```python
from build123d import *

# Parameters (mm, degrees)
CROQUIS2_W              = 180
CROQUIS2_H              = 90
SALIENTE_EXTRUIR1_DEPTH = 4
REDONDEO1_R             = 10
CORTAR_EXTRUIR1_REACH   = 102.703
CROQUIS8_R              = 2
CORTAR_EXTRUIR2_REACH   = 102.703
CROQUIS4_R              = 4
CROQUIS9_R              = 2
CORTAR_EXTRUIR3_DEPTH   = 101.702532242


with BuildPart() as part:
    # Croquis2 → Saliente-Extruir1 (new body)
    with BuildSketch(Plane(origin=(0, 0, 0), x_dir=(1, 0, 0), z_dir=(0, 1, 0))):
        Rectangle(CROQUIS2_W, CROQUIS2_H)
    extrude(amount=SALIENTE_EXTRUIR1_DEPTH)

    # Redondeo1
    redondeo1_edges = [part.edges().sort_by_distance(p)[0] for p in [
        (90, 2, 45),
        (-90, 2, 45),
        (-90, 2, -45),
        (90, 2, -45),
    ]]
    fillet(redondeo1_edges, radius=REDONDEO1_R)

    # Croquis8 → Cortar-Extruir1 (cut, up to next)
    with BuildSketch(Plane(origin=(0, 4, 0), x_dir=(1, 0, 0), z_dir=(0, 1, 0)), mode=Mode.PRIVATE) as cortar_extruir1_sk1:
        with Locations(Location((-47, 0, 0), (0, 0, 270))):
            Circle(CROQUIS8_R)
    cortar_extruir1_tool1 = extrude(cortar_extruir1_sk1.sketch, amount=-CORTAR_EXTRUIR1_REACH, mode=Mode.PRIVATE) & part.part
    # Croquis8 → Cortar-Extruir1 (cut, up to next)
    with BuildSketch(Plane(origin=(0, 4, 0), x_dir=(1, 0, 0), z_dir=(0, 1, 0)), mode=Mode.PRIVATE) as cortar_extruir1_sk2:
        with Locations(Location((-77, 0, 0), (0, 0, 270))):
            Circle(CROQUIS8_R)
    cortar_extruir1_tool2 = extrude(cortar_extruir1_sk2.sketch, amount=-CORTAR_EXTRUIR1_REACH, mode=Mode.PRIVATE) & part.part
    # Croquis8 → Cortar-Extruir1 (cut, up to next)
    with BuildSketch(Plane(origin=(0, 4, 0), x_dir=(1, 0, 0), z_dir=(0, 1, 0)), mode=Mode.PRIVATE) as cortar_extruir1_sk3:
        with Locations(Location((77, 0, 0), (0, 0, 90))):
            Circle(CROQUIS8_R)
    cortar_extruir1_tool3 = extrude(cortar_extruir1_sk3.sketch, amount=-CORTAR_EXTRUIR1_REACH, mode=Mode.PRIVATE) & part.part
    # Croquis8 → Cortar-Extruir1 (cut, up to next)
    with BuildSketch(Plane(origin=(0, 4, 0), x_dir=(1, 0, 0), z_dir=(0, 1, 0)), mode=Mode.PRIVATE) as cortar_extruir1_sk4:
        with Locations(Location((47, 0, 0), (0, 0, 90))):
            Circle(CROQUIS8_R)
    cortar_extruir1_tool4 = extrude(cortar_extruir1_sk4.sketch, amount=-CORTAR_EXTRUIR1_REACH, mode=Mode.PRIVATE) & part.part
    # Croquis8 → Cortar-Extruir1 (cut, up to next)
    with BuildSketch(Plane(origin=(0, 4, 0), x_dir=(1, 0, 0), z_dir=(0, 1, 0)), mode=Mode.PRIVATE) as cortar_extruir1_sk5:
        with Locations(Location((-77, 15.5, 0), (0, 0, 270))):
            Circle(CROQUIS8_R)
    cortar_extruir1_tool5 = extrude(cortar_extruir1_sk5.sketch, amount=-CORTAR_EXTRUIR1_REACH, mode=Mode.PRIVATE) & part.part
    # Croquis8 → Cortar-Extruir1 (cut, up to next)
    with BuildSketch(Plane(origin=(0, 4, 0), x_dir=(1, 0, 0), z_dir=(0, 1, 0)), mode=Mode.PRIVATE) as cortar_extruir1_sk6:
        with Locations(Location((-47, 15.5, 0), (0, 0, 270))):
            Circle(CROQUIS8_R)
    cortar_extruir1_tool6 = extrude(cortar_extruir1_sk6.sketch, amount=-CORTAR_EXTRUIR1_REACH, mode=Mode.PRIVATE) & part.part
    # Croquis8 → Cortar-Extruir1 (cut, up to next)
    with BuildSketch(Plane(origin=(0, 4, 0), x_dir=(1, 0, 0), z_dir=(0, 1, 0)), mode=Mode.PRIVATE) as cortar_extruir1_sk7:
        with Locations(Location((-77, -15.5, 0), (0, 0, 90))):
            Circle(CROQUIS8_R)
    cortar_extruir1_tool7 = extrude(cortar_extruir1_sk7.sketch, amount=-CORTAR_EXTRUIR1_REACH, mode=Mode.PRIVATE) & part.part
    # Croquis8 → Cortar-Extruir1 (cut, up to next)
    with BuildSketch(Plane(origin=(0, 4, 0), x_dir=(1, 0, 0), z_dir=(0, 1, 0)), mode=Mode.PRIVATE) as cortar_extruir1_sk8:
        with Locations(Location((-47, -15.5, 0), (0, 0, 90))):
            Circle(CROQUIS8_R)
    cortar_extruir1_tool8 = extrude(cortar_extruir1_sk8.sketch, amount=-CORTAR_EXTRUIR1_REACH, mode=Mode.PRIVATE) & part.part
    # Croquis8 → Cortar-Extruir1 (cut, up to next)
    with BuildSketch(Plane(origin=(0, 4, 0), x_dir=(1, 0, 0), z_dir=(0, 1, 0)), mode=Mode.PRIVATE) as cortar_extruir1_sk9:
        with Locations(Location((47, -15.5, 0), (0, 0, 270))):
            Circle(CROQUIS8_R)
    cortar_extruir1_tool9 = extrude(cortar_extruir1_sk9.sketch, amount=-CORTAR_EXTRUIR1_REACH, mode=Mode.PRIVATE) & part.part
    # Croquis8 → Cortar-Extruir1 (cut, up to next)
    with BuildSketch(Plane(origin=(0, 4, 0), x_dir=(1, 0, 0), z_dir=(0, 1, 0)), mode=Mode.PRIVATE) as cortar_extruir1_sk10:
        with Locations(Location((77, -15.5, 0), (0, 0, 270))):
            Circle(CROQUIS8_R)
    cortar_extruir1_tool10 = extrude(cortar_extruir1_sk10.sketch, amount=-CORTAR_EXTRUIR1_REACH, mode=Mode.PRIVATE) & part.part
    # Croquis8 → Cortar-Extruir1 (cut, up to next)
    with BuildSketch(Plane(origin=(0, 4, 0), x_dir=(1, 0, 0), z_dir=(0, 1, 0)), mode=Mode.PRIVATE) as cortar_extruir1_sk11:
        with Locations(Location((77, 15.5, 0), (0, 0, 90))):
            Circle(CROQUIS8_R)
    cortar_extruir1_tool11 = extrude(cortar_extruir1_sk11.sketch, amount=-CORTAR_EXTRUIR1_REACH, mode=Mode.PRIVATE) & part.part
    # Croquis8 → Cortar-Extruir1 (cut, up to next)
    with BuildSketch(Plane(origin=(0, 4, 0), x_dir=(1, 0, 0), z_dir=(0, 1, 0)), mode=Mode.PRIVATE) as cortar_extruir1_sk12:
        with Locations(Location((47, 15.5, 0), (0, 0, 90))):
            Circle(CROQUIS8_R)
    cortar_extruir1_tool12 = extrude(cortar_extruir1_sk12.sketch, amount=-CORTAR_EXTRUIR1_REACH, mode=Mode.PRIVATE) & part.part
    add(cortar_extruir1_tool1.solids().sort_by_distance((-47, 4, 0))[0], mode=Mode.SUBTRACT)
    add(cortar_extruir1_tool2.solids().sort_by_distance((-77, 4, 0))[0], mode=Mode.SUBTRACT)
    add(cortar_extruir1_tool3.solids().sort_by_distance((77, 4, 0))[0], mode=Mode.SUBTRACT)
    add(cortar_extruir1_tool4.solids().sort_by_distance((47, 4, 0))[0], mode=Mode.SUBTRACT)
    add(cortar_extruir1_tool5.solids().sort_by_distance((-77, 4, -15.5))[0], mode=Mode.SUBTRACT)
    add(cortar_extruir1_tool6.solids().sort_by_distance((-47, 4, -15.5))[0], mode=Mode.SUBTRACT)
    add(cortar_extruir1_tool7.solids().sort_by_distance((-77, 4, 15.5))[0], mode=Mode.SUBTRACT)
    add(cortar_extruir1_tool8.solids().sort_by_distance((-47, 4, 15.5))[0], mode=Mode.SUBTRACT)
    add(cortar_extruir1_tool9.solids().sort_by_distance((47, 4, 15.5))[0], mode=Mode.SUBTRACT)
    add(cortar_extruir1_tool10.solids().sort_by_distance((77, 4, 15.5))[0], mode=Mode.SUBTRACT)
    add(cortar_extruir1_tool11.solids().sort_by_distance((77, 4, -15.5))[0], mode=Mode.SUBTRACT)
    add(cortar_extruir1_tool12.solids().sort_by_distance((47, 4, -15.5))[0], mode=Mode.SUBTRACT)

    # Croquis4 → Cortar-Extruir2 (cut, up to next)
    with BuildSketch(Plane(origin=(0, 4, 0), x_dir=(1, 0, 0), z_dir=(0, 1, 0)), mode=Mode.PRIVATE) as cortar_extruir2_sk1:
        with Locations(Location((-80, 35, 0), (0, 0, 270))):
            Circle(CROQUIS4_R)
    cortar_extruir2_tool1 = extrude(cortar_extruir2_sk1.sketch, amount=-CORTAR_EXTRUIR2_REACH, mode=Mode.PRIVATE) & part.part
    # Croquis4 → Cortar-Extruir2 (cut, up to next)
    with BuildSketch(Plane(origin=(0, 4, 0), x_dir=(1, 0, 0), z_dir=(0, 1, 0)), mode=Mode.PRIVATE) as cortar_extruir2_sk2:
        with Locations(Location((-80, -35, 0), (0, 0, 270))):
            Circle(CROQUIS4_R)
    cortar_extruir2_tool2 = extrude(cortar_extruir2_sk2.sketch, amount=-CORTAR_EXTRUIR2_REACH, mode=Mode.PRIVATE) & part.part
    # Croquis4 → Cortar-Extruir2 (cut, up to next)
    with BuildSketch(Plane(origin=(0, 4, 0), x_dir=(1, 0, 0), z_dir=(0, 1, 0)), mode=Mode.PRIVATE) as cortar_extruir2_sk3:
        with Locations(Location((80, -35, 0), (0, 0, 90))):
            Circle(CROQUIS4_R)
    cortar_extruir2_tool3 = extrude(cortar_extruir2_sk3.sketch, amount=-CORTAR_EXTRUIR2_REACH, mode=Mode.PRIVATE) & part.part
    # Croquis4 → Cortar-Extruir2 (cut, up to next)
    with BuildSketch(Plane(origin=(0, 4, 0), x_dir=(1, 0, 0), z_dir=(0, 1, 0)), mode=Mode.PRIVATE) as cortar_extruir2_sk4:
        with Locations(Location((80, 35, 0), (0, 0, 90))):
            Circle(CROQUIS4_R)
    cortar_extruir2_tool4 = extrude(cortar_extruir2_sk4.sketch, amount=-CORTAR_EXTRUIR2_REACH, mode=Mode.PRIVATE) & part.part
    add(cortar_extruir2_tool1.solids().sort_by_distance((-80, 4, -35))[0], mode=Mode.SUBTRACT)
    add(cortar_extruir2_tool2.solids().sort_by_distance((-80, 4, 35))[0], mode=Mode.SUBTRACT)
    add(cortar_extruir2_tool3.solids().sort_by_distance((80, 4, 35))[0], mode=Mode.SUBTRACT)
    add(cortar_extruir2_tool4.solids().sort_by_distance((80, 4, -35))[0], mode=Mode.SUBTRACT)

    # Croquis9 → Cortar-Extruir3 (cut, through all)
    with BuildSketch(Plane(origin=(0, 4, 0), x_dir=(1, 0, 0), z_dir=(0, 1, 0))):
        with Locations(Location((0, 28, 0), (0, 0, 270))):
            Circle(CROQUIS9_R)
        with Locations(Location((-28, 0, 0), (0, 0, 270))):
            Circle(CROQUIS9_R)
        with Locations(Location((0, -28, 0), (0, 0, 90))):
            Circle(CROQUIS9_R)
        with Locations(Location((28, 0, 0), (0, 0, 90))):
            Circle(CROQUIS9_R)
    extrude(amount=-CORTAR_EXTRUIR3_DEPTH, mode=Mode.SUBTRACT)


solid = part.part
```
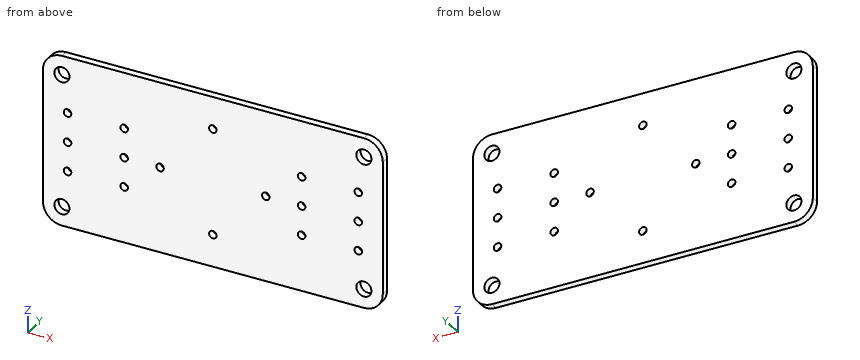
Build history of the part. All positions in model axes, mm. Give positions to 0.01 mm unless a question says otherwise; leave off trailing zeros. Loops run counter-clockwise (first coordinate to the right, second up) from the corner with the lowest first, then second, coordinate; pieces in that order, holes last.
Item 1: Slice it at A-A, the plane z = 28. List the corners of the cut face in (x, y).
Answers follow:
outline: (-90, 0) - (-2, 0) - (-2, 4) - (-90, 4) - close; (2, 0) - (90, 0) - (90, 4) - (2, 4) - close
Item 2: Drill centre lines: line 1 (Z direction, x = 80, y = 1.45); line 2 (X direction, y = 2.85, z = 15.5); line 3 (X direction, y = 1.5, z = 35.5). Where is each one in solid material? Low to high.
Answers follow:
line 1: z = -45 to -39, -31 to 31, 39 to 45
line 2: x = -90 to -79, -75 to -49, -45 to 45, 49 to 75, 79 to 90
line 3: x = -89.99 to -83.97, -76.03 to 76.03, 83.97 to 89.99
Item 3: Slice it at B-B, the plane x = 0. List the corners of the cut face in (y, z).
Answers follow:
outline: (0, -45) - (4, -45) - (4, -30) - (0, -30) - close; (0, -26) - (4, -26) - (4, 26) - (0, 26) - close; (0, 30) - (4, 30) - (4, 45) - (0, 45) - close
Item 4: Slice it at C-C, the plane z = 15.5. List the corners of the cut face in (x, y), and give its area (3 significant figures).
Answers follow:
outline: (-90, 0) - (-79, 0) - (-79, 4) - (-90, 4) - close; (-75, 0) - (-49, 0) - (-49, 4) - (-75, 4) - close; (-45, 0) - (45, 0) - (45, 4) - (-45, 4) - close; (49, 0) - (75, 0) - (75, 4) - (49, 4) - close; (79, 0) - (90, 0) - (90, 4) - (79, 4) - close
area: 656 mm2
Item 5: Slice it at D-D, the plane x = 28. List the corners of the cut face in (y, z), and give its area (3 significant figures).
Answers follow:
outline: (0, -45) - (4, -45) - (4, -2) - (0, -2) - close; (0, 2) - (4, 2) - (4, 45) - (0, 45) - close
area: 344 mm2
